Read the model definition and answer for the solid it produces. Units are mm, in the model's axes. A direction names the side the tool comes from. Give positions to 0.01 mm unless a question says otherwise; leave off trailing zeros. Order: outer loops, then holes, each group sorted by start corner. A loop starts at its lowest first (then second) coordinate and runs counter-clockwise, first axis right, second up. Notation, with made-up numbers: (58, -17) - (93, -17) arc R17 cw to (93, 10) - close; hole circle Ø9 at (-30, 20.5). An arc over 180 degrees is marked (long way). Write each question's results on one line, items separated by ' | '. Start each with the question number.
Q1. Find section A-A on y = 18.5. Give the vertices of the cut face in (x, z).
Q2. Find section C-C on y = 39.5. Give the vertices of the cut face in (x, z), and give its area (3 significant figures).
Q3. Find section B-B on z = 33.5. Give the vertices of the cut face in (x, y).
Q4. Find the intervals of material crossed by line 1 along X through (y, z) = (-47, 16); line 2 along Y through (x, z) = (36, 5); line 3 along X through (y, z) = (-31.5, 7), in increasing order. Write a range as from..to.
Q5. For a pull along Y with two mould halves and no side action, classify faces 6 (the face through (92, -1, 2)), 7 (the face through (-1, 51.5, 8)), 8 (the face through (104, -41.6, 48.8)) as +Y half, -Y half, draft (parallel to the pull), parting line (faces both ways), or undercut.
Q6. A tool of negligible diameter and unlimited length cuts with its end or side. For faces 1 (the face through (-95.535, -39.863, 54.444)), 2 (the face through (95.465, -39.863, 54.444)), 3 (the face through (-85, -1, 15)), 4 (the face through (76.65, -14.2, 91.64)), 5 (the face through (-78, -46, 12)), from which of +Z, -Z, +X, -X, +Y, -Y can it reach the whole face along a straight path? Write none if from no direction.
Q7. Flat-ended cylindrical pins translate along their axes: P1, Ø22.5, axis at x = -72.5, y = -41.5, coming from the -Z side; P2, Ø10, axis at x = 11.5, z = 40, coming from the -Y side; P3, Ø16.5, axis at y = -18, z = 10.5, coming from the +X side; P4, Ø1.5, axis at x = 28.5, z = 32, coming from the +Y side. Find the tip coordinate at first contact, or state that the pin passes through.
from build123d import *

# Parameters (mm, degrees)
SKETCH1_W                = 173
SKETCH1_H                = 109
SKETCH1_W_2              = 167
SKETCH1_H_2              = 103
EXTRUDE_THIN1_DEPTH      = 15
BOSS_EXTRUDE1_DEPTH      = 3
BOSS_EXTRUDE2_DEPTH      = 86.5
BOSS_EXTRUDE2_DEPTH_BACK = 86.5
MOVE_START               = 86.5
MOVE_FACE1_DEPTH         = 6.5
MOVE_START_2             = -93
MOVE_FACE2_DEPTH         = 6.5
BOSS_EXTRUDE3_START      = -93
BOSS_EXTRUDE3_DEPTH      = 186
BOSS_EXTRUDE3_2_DEPTH    = 3
BOSS_EXTRUDE3_START_2    = 90
BOSS_EXTRUDE3_3_DEPTH    = 3
FILLET3_R                = 100
FILLET2_R                = 2
SKETCH8_R                = 2.5
BOSS_EXTRUDE4_DEPTH      = 10
SKETCH8_3_R              = 2.5
CUT_EXTRUDE1_DEPTH       = 6
SKETCH9_R                = 2.25
BOSS_EXTRUDE5_DEPTH      = 5
FILLET4_R                = 5


# Read off the part's stored shape, not the designer's step: Move Face1, Move Face2, Boss-Extrude3
with BuildPart() as part:
    # Sketch1 → Extrude-Thin1 (new body)
    with BuildSketch(Plane.XY):
        Rectangle(SKETCH1_W, SKETCH1_H)
        Rectangle(SKETCH1_W_2, SKETCH1_H_2, mode=Mode.SUBTRACT)
    extrude(amount=EXTRUDE_THIN1_DEPTH)

    # Sketch2 → Boss-Extrude1 (add)
    with BuildSketch(Plane.XY.offset(15)):
        Polygon((63.701010127, 51.5), (83.5, 31.701010127), (83.5, 51.5), align=None)
        Polygon((-83.5, 51.5), (-83.5, 31.701010127), (-63.701010127, 51.5), align=None)
        Polygon((83.5, -31.701010127), (63.701010127, -51.5), (83.5, -51.5), align=None)
        Polygon((-83.5, -31.701010127), (-83.5, -51.5), (-63.701010127, -51.5), align=None)
    extrude(amount=-BOSS_EXTRUDE1_DEPTH)

    # Sketch5 → Boss-Extrude2 (add, two sides: drawn at the far end of the back side and taken through both)
    with BuildSketch(Plane(origin=(0, 0, 0), x_dir=(0, 0, -1), z_dir=(1, 0, 0)).offset(-BOSS_EXTRUDE2_DEPTH_BACK)):
        with BuildLine():
            Line((-15, -54.5), (-8.784019086, -56.400416081))
            add(Edge.make_bspline(
                [(0, -54.5), (-2.80635361, -54.592909142), (-6.451217818, -54.49036495), (-8.784019086, -56.400416081)],
                knots=[0, 0, 0, 0, 1, 1, 1, 1], degree=3))
            Line((0, -54.5), (-15, -54.5))
        make_face()
    extrude(amount=BOSS_EXTRUDE2_DEPTH + BOSS_EXTRUDE2_DEPTH_BACK)

    # Move Face1 outline → Move Face1 (add)
    with BuildSketch(Plane.YZ.offset(MOVE_START)):
        with BuildLine():
            Line((-54.5, 15), (-56.400416081, 8.784019086))
            add(Edge.make_bspline(
                [(-56.400416081, 8.784019086), (-54.49036495, 6.451217818), (-54.592909142, 2.80635361), (-54.5, 0)],
                knots=[0, 0, 0, 0, 1, 1, 1, 1], degree=3))
            Line((-54.5, 0), (54.5, 0))
            Line((54.5, 0), (54.5, 15))
            Line((54.5, 15), (-54.5, 15))
        make_face()
    extrude(amount=MOVE_FACE1_DEPTH)

    # Move Face2 outline → Move Face2 (add)
    with BuildSketch(Plane.YZ.offset(MOVE_START_2)):
        with BuildLine():
            Line((-54.5, 15), (-56.400416081, 8.784019086))
            add(Edge.make_bspline(
                [(-56.400416081, 8.784019086), (-54.49036495, 6.451217818), (-54.592909142, 2.80635361), (-54.5, 0)],
                knots=[0, 0, 0, 0, 1, 1, 1, 1], degree=3))
            Line((-54.5, 0), (54.5, 0))
            Line((54.5, 0), (54.5, 15))
            Line((54.5, 15), (-54.5, 15))
        make_face()
    extrude(amount=MOVE_FACE2_DEPTH)

    # Boss-Extrude3 outline → Boss-Extrude3 (add)
    with BuildSketch(Plane.YZ.offset(BOSS_EXTRUDE3_START)):
        Polygon((-28.186546575, 101.067428037), (-54.5, 15), (-51.362924731, 15), (-25.317632307, 100.190312923), align=None)
        Polygon((71.496001129, 70.591414798), (68.627086861, 71.468529912), (51.362924731, 15), (54.5, 15), align=None)
    extrude(amount=BOSS_EXTRUDE3_DEPTH)

    # Boss-Extrude3 2 outline → Boss-Extrude3 2 (add)
    with BuildSketch(Plane.YZ.offset(BOSS_EXTRUDE3_START)):
        Polygon((68.627086861, 71.468529912), (-25.317632307, 100.190312923), (-51.362924731, 15), (51.362924731, 15), align=None)
    extrude(amount=BOSS_EXTRUDE3_2_DEPTH)

    # Boss-Extrude3 3 outline → Boss-Extrude3 3 (add)
    with BuildSketch(Plane.YZ.offset(BOSS_EXTRUDE3_START_2)):
        Polygon((68.627086861, 71.468529912), (-25.317632307, 100.190312923), (-51.362924731, 15), (51.362924731, 15), align=None)
    extrude(amount=BOSS_EXTRUDE3_3_DEPTH)

    # Fillet3
    fillet3_edges = [part.edges().sort_by_distance(p)[0] for p in [
        (0, 54.5, 15),
    ]]
    fillet(fillet3_edges, radius=FILLET3_R)

    # Fillet2
    # the kernel refuses this fillet: 2 mm, written as the material it adds along each edge
    with BuildSketch(Plane(origin=(83.5, 31.701010127, 15), x_dir=(0, -1, 0), z_dir=(0, 0, -1)), Plane(origin=(-63.701010127, 51.5, 15), x_dir=(1, 0, 0), z_dir=(0, 0, -1)), Plane(origin=(63.701010127, -51.5, 15), x_dir=(-1, 0, 0), z_dir=(0, 0, -1)), Plane(origin=(-83.5, -31.701010127, 15), x_dir=(0, 1, 0), z_dir=(0, 0, -1))) as fillet2_piece_1:
        with BuildLine():
            CenterArc((FILLET2_R * 0.414213562373, FILLET2_R), FILLET2_R, 225, 45)
            Line((-FILLET2_R * 0.292893218813, FILLET2_R * 0.292893218813), (0, 0))
            Line((0, 0), (FILLET2_R * 0.414213562373, 0))
        make_face()
    extrude(amount=3)
    with BuildSketch(Plane(origin=(63.701010127, 51.5, 15), x_dir=(-1, 0, 0), z_dir=(0, 0, -1)), Plane(origin=(-83.5, 31.701010127, 15), x_dir=(0, -1, 0), z_dir=(0, 0, -1)), Plane(origin=(83.5, -31.701010127, 15), x_dir=(0, 1, 0), z_dir=(0, 0, -1)), Plane(origin=(-63.701010127, -51.5, 15), x_dir=(1, 0, 0), z_dir=(0, 0, -1))) as fillet2_piece_2:
        with BuildLine():
            CenterArc((FILLET2_R * 0.414213562373, -FILLET2_R), FILLET2_R, 90, 45)
            Line((-FILLET2_R * 0.292893218813, -FILLET2_R * 0.292893218813), (0, 0))
            Line((0, 0), (FILLET2_R * 0.414213562373, 0))
        make_face()
    extrude(amount=3)

    # Sketch8 → Boss-Extrude4 (add)
    # profile 1 of 8: a face of its own
    with BuildSketch(Plane(origin=(0, 25.848674053, 84.547203211), x_dir=(1, 0, 0), z_dir=(0, 0.2923717047227412, 0.9563047559630341))):
        Polygon((-90, 19.714270268), (-63.838085396, 44.733033629), (-90, 44.733033629), align=None)
        with Locations((-83.459521349, 38.478342789)):
            Circle(SKETCH8_R, mode=Mode.SUBTRACT)
    # profile 2 of 8: a face of its own
    with BuildSketch(Plane(origin=(0, 25.848674053, 84.547203211), x_dir=(1, 0, 0), z_dir=(0, 0.2923717047227412, 0.9563047559630341))):
        with Locations((-83.459521349, 38.478342789)):
            Circle(SKETCH8_R)
    # profile 3 of 8: a face of its own
    with BuildSketch(Plane(origin=(0, 25.848674053, 84.547203211), x_dir=(1, 0, 0), z_dir=(0, 0.2923717047227412, 0.9563047559630341))):
        Polygon((62.943139485, -53.504184771), (90, -53.504184771), (90, -27.608306296), (62.920893352, -53.504184771), align=None)
        with Locations((83.230223338, -47.030215152)):
            Circle(SKETCH8_R, mode=Mode.SUBTRACT)
    # profile 4 of 8: a face of its own
    with BuildSketch(Plane(origin=(0, 25.848674053, 84.547203211), x_dir=(1, 0, 0), z_dir=(0, 0.2923717047227412, 0.9563047559630341))):
        with Locations((83.230223338, -47.030215152)):
            Circle(SKETCH8_R)
    # profile 5 of 8: a face of its own
    with BuildSketch(Plane(origin=(0, 25.848674053, 84.547203211), x_dir=(1, 0, 0), z_dir=(0, 0.2923717047227412, 0.9563047559630341))):
        Polygon((-90, -53.504184771), (-62.920893352, -53.504184771), (-90, -27.608306296), align=None)
        with Locations((-83.230223338, -47.030215152)):
            Circle(SKETCH8_R, mode=Mode.SUBTRACT)
    # profile 6 of 8: a face of its own
    with BuildSketch(Plane(origin=(0, 25.848674053, 84.547203211), x_dir=(1, 0, 0), z_dir=(0, 0.2923717047227412, 0.9563047559630341))):
        with Locations((-83.230223338, -47.030215152)):
            Circle(SKETCH8_R)
    # profile 7 of 8: a face of its own
    with BuildSketch(Plane(origin=(0, 25.848674053, 84.547203211), x_dir=(1, 0, 0), z_dir=(0, 0.2923717047227412, 0.9563047559630341))):
        Polygon((63.838085396, 44.733033629), (90, 19.714270268), (90, 44.733033629), align=None)
        with Locations((83.459521349, 38.478342789)):
            Circle(SKETCH8_R, mode=Mode.SUBTRACT)
    # profile 8 of 8: a face of its own
    with BuildSketch(Plane(origin=(0, 25.848674053, 84.547203211), x_dir=(1, 0, 0), z_dir=(0, 0.2923717047227412, 0.9563047559630341))):
        with Locations((83.459521349, 38.478342789)):
            Circle(SKETCH8_R)
    extrude(amount=-BOSS_EXTRUDE4_DEPTH)

    # Sketch8<3> → Cut-Extrude1 (cut)
    with BuildSketch(Plane(origin=(0, 25.848674053, 84.547203211), x_dir=(1, 0, 0), z_dir=(0, 0.2923717047227412, 0.9563047559630341))):
        with Locations(Location((-83.459521349, 38.478342789, 0), (0, 0, 270))):
            Circle(SKETCH8_3_R)
        with Locations(Location((83.459521349, 38.478342789, 0), (0, 0, 270))):
            Circle(SKETCH8_3_R)
        with Locations(Location((-83.230223338, -47.030215152, 0), (0, 0, 270))):
            Circle(SKETCH8_3_R)
        with Locations(Location((83.230223338, -47.030215152, 0), (0, 0, 270))):
            Circle(SKETCH8_3_R)
    extrude(amount=-CUT_EXTRUDE1_DEPTH, mode=Mode.SUBTRACT)

    # Sketch9 → Boss-Extrude5 (add)
    # profile 1 of 2: a face of its own
    with BuildSketch(Plane(origin=(0, -54.035220628, 16.520224825), x_dir=(1, 0, 0), z_dir=(0, -0.956304755963037, 0.29237170472273216))):
        with BuildLine():
            Line((-98, 40.410313432), (-93, 40.410313432))
            Line((-93, 40.410313432), (-93, 28.410313432))
            Line((-93, 28.410313432), (-98, 28.410313432))
            ThreePointArc((-98, 28.410313432), (-104, 34.410313432), (-98, 40.410313432))
        make_face()
        with Locations(Location((-98, 34.410313432, 0), (0, 0, 270))):
            Circle(SKETCH9_R, mode=Mode.SUBTRACT)
    # profile 2 of 2: a face of its own
    with BuildSketch(Plane(origin=(0, -54.035220628, 16.520224825), x_dir=(1, 0, 0), z_dir=(0, -0.956304755963037, 0.29237170472273216))):
        with BuildLine():
            Line((93, 40.410313432), (98, 40.410313432))
            ThreePointArc((98, 40.410313432), (104, 34.410313432), (98, 28.410313432))
            Line((98, 28.410313432), (93, 28.410313432))
            Line((93, 28.410313432), (93, 40.410313432))
        make_face()
        with Locations(Location((98, 34.410313432, 0), (0, 0, 270))):
            Circle(SKETCH9_R, mode=Mode.SUBTRACT)
    extrude(amount=-BOSS_EXTRUDE5_DEPTH)

    # Fillet4
    # the kernel refuses this fillet: 5 mm, written as the material it takes off along each edge
    with BuildSketch(Plane(origin=(-93, -67, 0), x_dir=(1, 0, 0), z_dir=(0, 1, 0))) as fillet4_piece_1:
        with BuildLine():
            CenterArc((FILLET4_R, -FILLET4_R), FILLET4_R, 90, 90)
            Line((0, -FILLET4_R), (-FILLET4_R * 0.02, -FILLET4_R))
            Line((-FILLET4_R * 0.02, -FILLET4_R), (-FILLET4_R * 0.02, FILLET4_R * 0.02))
            Line((-FILLET4_R * 0.02, FILLET4_R * 0.02), (FILLET4_R, FILLET4_R * 0.02))
            Line((FILLET4_R, FILLET4_R * 0.02), (FILLET4_R, 0))
        make_face()
    extrude(amount=134, mode=Mode.SUBTRACT)
    with BuildSketch(Plane(origin=(86.5, -54.5, 0), x_dir=(0, 1, 0), z_dir=(-1, 0, 0)), Plane(origin=(0, -54.5, 0), x_dir=(0, 1, 0), z_dir=(-1, 0, 0))) as fillet4_piece_2:
        with BuildLine():
            CenterArc((4.719023174, -5), FILLET4_R, 90, 82.540825882)
            Line((-0.238664904, -4.350901455), (-0.337818666, -4.337919484))
            ThreePointArc((-0.337818666, -4.337919484), (-0.165294679, -2.173525325), (-0.099945242, 0.003308858))
            Line((-0.099945242, 0.003308858), (0, 0.1))
            Line((0, 0.1), (4.719023174, 0.1))
            Line((4.719023174, 0.1), (4.719023174, 0))
        make_face()
    extrude(amount=86.5, mode=Mode.SUBTRACT)
    with BuildSketch(Plane(origin=(105.208719161, 54.5, 0), x_dir=(0, -1, 0), z_dir=(-1, 0, 0))) as fillet4_piece_3:
        with BuildLine():
            CenterArc((4.883487664, 5), FILLET4_R, 182.699411552, 87.300588448)
            Line((-0.110964129, 4.764519041), (-0.610409308, 4.740970945))
            ThreePointArc((-0.610409308, 4.740970945), (-0.5, 0.054899865), (-0.5, 0))
            Line((-0.5, 0), (0, -0.5))
            Line((0, -0.5), (4.883487664, -0.5))
            Line((4.883487664, -0.5), (4.883487664, 0))
        make_face()
    extrude(amount=210.417438322, mode=Mode.SUBTRACT)
    with BuildSketch(Plane(origin=(93, -67, 0), x_dir=(-1, 0, 0), z_dir=(0, 1, 0))) as fillet4_piece_4:
        with BuildLine():
            CenterArc((FILLET4_R, FILLET4_R), FILLET4_R, 180, 90)
            Line((0, FILLET4_R), (-FILLET4_R * 0.02, FILLET4_R))
            Line((-FILLET4_R * 0.02, FILLET4_R), (-FILLET4_R * 0.02, -FILLET4_R * 0.02))
            Line((-FILLET4_R * 0.02, -FILLET4_R * 0.02), (FILLET4_R, -FILLET4_R * 0.02))
            Line((FILLET4_R, -FILLET4_R * 0.02), (FILLET4_R, 0))
        make_face()
    extrude(amount=134, mode=Mode.SUBTRACT)
    with BuildSketch(Plane(origin=(86.5, -54.5, 0), x_dir=(0, 1, 0), z_dir=(1, 0, 0)), Plane(origin=(-104.797557934, -54.5, 0), x_dir=(0, 1, 0), z_dir=(1, 0, 0))) as fillet4_piece_5:
        with BuildLine():
            CenterArc((4.719023174, 5), FILLET4_R, 187.459174119, 82.540825881)
            Line((-0.238664904, 4.350901455), (-0.337818666, 4.337919484))
            ThreePointArc((-0.337818666, 4.337919484), (-0.165294679, 2.173525325), (-0.099945242, -0.003308858))
            Line((-0.099945242, -0.003308858), (0, -0.1))
            Line((0, -0.1), (4.719023174, -0.1))
            Line((4.719023174, -0.1), (4.719023174, 0))
        make_face()
    extrude(amount=18.297557934, mode=Mode.SUBTRACT)


solid = part.part
Working result:
1) outline: (-93, 5) arc R5 ccw to (-88, 0) - (-83.5, 0) - (-83.5, 15) - (-90, 15) - (-90, 86.79) - (-93, 86.79) - close; (83.5, 0) - (88, 0) arc R5 ccw to (93, 5) - (93, 86.79) - (90, 86.79) - (90, 15) - (83.5, 15) - close
2) outline: (-93, 5) arc R5 ccw to (-88, 0) - (-83.5, 0) - (-83.5, 12) - (-75.7, 12) - (-75.7, 15) - (-90, 15) - (-90, 80.37) - (-93, 80.37) - close; (75.7, 12) - (83.5, 12) - (83.5, 0) - (88, 0) arc R5 ccw to (93, 5) - (93, 80.37) - (90, 80.37) - (90, 15) - (75.7, 15) - close | area: 713 mm²
3) outline: (-93, -48.84) - (93, -48.84) - (93, 60.16) - (-93, 60.16) - close; hole (-90, -45.71) - (90, -45.71) - (90, 57.02) - (-90, 57.02) - close
4) line 1: -93..-90, 90..93 | line 2: -54.84..-51.5, 51.5..54.62 | line 3: -93..-83.5, 83.5..93
5) face 6: draft | face 7: undercut | face 8: parting line
6) face 1: +Z, -X, +Y | face 2: +Z, +X, +Y | face 3: none | face 4: +Y | face 5: -Z
7) P1: z = 0 | P2: y = -48.39 | P3: x = 93 | P4: y = 59.93
